Autodesk Inventor part; units mm, degrees
ref_plane "YZ Plane" through (0, 0, 0) normal (1, 0, 0) x (0, 1, 0)
ref_plane "XZ Plane" through (0, 0, 0) normal (0, 1, 0) x (-1, 0, 0)
ref_plane "XY Plane" through (0, 0, 0) normal (0, 0, 1) x (1, 0, 0)
sketch "Sketch1" plane through (0, 0, 0) normal (0, 1, 0) x (-1, 0, 0)
  line L0 (0, 0) -> (110, 0)
  line L1 (110, 0) -> (110, -110)
  line L2 (110, -110) -> (0, -110)
  line L3 (0, -110) -> (0, 0)
  dimension "d0" = 110
  dimension "d1" = 110
extrude "Extrusion1" add sketch "Sketch1" along normal blind 10
sketch "Sketch2" plane through (0, 10, 0) normal (0, 1, 0) x (1, 0, 0)
  circle A0 centre (-85, 85) radius 6
  line L0 (-110, 110) -> (-110, 0)
  line L1 (0, 110) -> (-110, 110)
  line L2 (0, 0) -> (0, 110)
  line L3 (-110, 0) -> (0, 0)
  dimension "d11" = 12
  dimension "d12" = 25
  dimension "d13" = 25
extrude "Extrusion3" add sketch "Sketch2" along normal blind 75 contours A0
chamfer "Chamfer1" distance 3 angle 45 1 edges at (-91, 85, -85)
properties part number "base"
Work out the finished part from the listing and answer in its coordinate system (mm). A direction names the side the tool comes from. Coordinates: 2 decimals unless noted, no trailing zeros. Write each loop counter-clockwise with the first axis right and the second up, starting at its lowest first coordinate (ties: lowest second). Pieces come first, ordered by that corner, then holes.
Q1. A cutting plane is placed at B-B, the plane z = -85. Give the vertices of the cut face in (x, y), then the cut area to 3 significant figures.
Q2. A cutting plane is placed at A-A, the plane x = -85. Give the vertices of the cut face in (y, z).
Q3. Which of the six approach directions +Z, -Z, +X, -X, +Y, -Y give full straight-line access (tool end or side, diameter ignored) to faces 1 (the face through (-56, 5, -110)), 2 (the face through (-89.42, 45.5, -80.94))?
Q4. A cutting plane is placed at D-D, the plane x = -66. Give the vertices of the cut face in (y, z), then the cut area to 3 significant figures.
Q5. Find the intervals of material crossed by line 1 (Y direction, x = -35, z = -44.5); line 2 (Z direction, x = -81.5, y = 60.5); line 3 (Y direction, x = -85, z = -88.5), in increasing order.
Q6. A cutting plane is placed at C-C, the plane y = 13.5. Give the vertices of the cut face in (x, z).
Q7. Each of these flat-tipped pins is pushed along its axis until it touches: pin 1 Ø10 at (y, z) = (39, -78) entering from +X; pin 2 Ø12 at (x, z) = (-61.5, -93.5) entering from +Y. Where does it stop, or does it pass through?
Findings below:
1. outline: (-110, 0) - (0, 0) - (0, 10) - (-79, 10) - (-79, 82) - (-82, 85) - (-88, 85) - (-91, 82) - (-91, 10) - (-110, 10) - close
1. area: 1,990 mm2
2. outline: (0, -110) - (10, -110) - (10, -91) - (82, -91) - (85, -88) - (85, -82) - (82, -79) - (10, -79) - (10, 0) - (0, 0) - close
3. face 1: -Z, +X, -X, +Y, -Y
3. face 2: +Y
4. outline: (0, -110) - (10, -110) - (10, 0) - (0, 0) - close
4. area: 1,100 mm2
5. line 1: y = 0 to 10
5. line 2: z = -89.87 to -80.13
5. line 3: y = 0 to 84.5
6. outline: circle Ø12 at (-85, -85)
7. pin 1: stops at x = -79.34
7. pin 2: stops at y = 10
